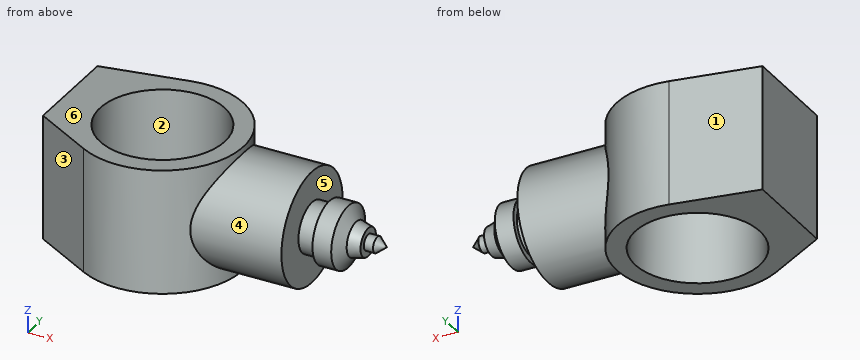
from build123d import *

# Parameters (mm, degrees)
IZIM1_R                          = 50
Y_KSEKLIK_EKSTR_ZYON1_DEPTH      = 50
Y_KSEKLIK_EKSTR_ZYON2_REACH      = 218.16
Y_KSEKLIK_EKSTR_ZYON2_END_RADIUS = 65
IZIM2_R                          = 45


with BuildPart() as part:
    # Çizim1 → Yükseklik-Ekstrüzyon1 (new, symmetric)
    with BuildSketch(Plane.XY):
        with BuildLine():
            Line((-80, -28.89070525), (-80, 51.10929475))
            Line((-80, 51.10929475), (-12, 63.882705015))
            ThreePointArc((-12, 63.882705015), (64.076421536, -10.918434095), (-32.479384713, -56.303548455))
            Line((-32.479384713, -56.303548455), (-80, -28.89070525))
        make_face()
        Circle(IZIM1_R, mode=Mode.SUBTRACT)
    extrude(amount=Y_KSEKLIK_EKSTR_ZYON1_DEPTH, both=True)

    # Yükseklik-Ekstrüzyon2: up to this cylinder (the profile starts outside it)
    y_kseklik_ekstr_zyon2_end = Plane(origin=(0, 0, 0), z_dir=(0, 0, -1)) * Cylinder(Y_KSEKLIK_EKSTR_ZYON2_END_RADIUS, 567.32, mode=Mode.PRIVATE)
    # Çizim2 → Yükseklik-Ekstrüzyon2 (add, up to the surface)
    with BuildSketch(Plane(origin=(120, 0, 0), x_dir=(0, 0, -1), z_dir=(1, 0, 0)), mode=Mode.PRIVATE) as y_kseklik_ekstr_zyon2_sk1:
        Circle(IZIM2_R)
    y_kseklik_ekstr_zyon2_tool1 = extrude(y_kseklik_ekstr_zyon2_sk1.sketch, amount=-Y_KSEKLIK_EKSTR_ZYON2_REACH, mode=Mode.PRIVATE) - y_kseklik_ekstr_zyon2_end
    add(y_kseklik_ekstr_zyon2_tool1.solids().sort_by_distance((120, 0, 0))[0])

    # Çizim3 → Döndür1 (revolve)
    with BuildSketch(Plane.XY, mode=Mode.PRIVATE) as d_nd_r1_sk:
        Polygon((164.385328123, -6.351150209), (172.385328123, -6.351150209), (180.109503873, 0), (120, 0), (120, -20), (134, -20), (134, -25), (149, -25), (155.385874648, -13.93934066), (165.04513291, -11.351150209), (165.04513291, -6.351150209), align=None)
    revolve(d_nd_r1_sk.sketch.rotate(Axis((0, 0, 0), (1, 0, 0)), 270), axis=Axis((0, 0, 0), (1, 0, 0)))


solid = part.part
Input: part model. Units: mm. Frame: model coordinates. Face numbers are marked on the shaded views. A direction names the side the tool comes from. Coordinates: 2 decimals unless noted, no trailing zeros. Order: outer loops, then holes, each group sorted by start corner. A loop starts at its lowest first (then second) coordinate and runs counter-clockwise, first axis right, second up. Notation, with made-up numbers: M 3,-39 L 37,-39 A22 cw 37,-33 Z; hole C -14,-33.5 d5. An arc over 180 degrees is marked long. Answer in a Markdown table with one row per item.
(1) Contact query for flat-ended pins moving along their axis: pin 1 Ø5 at (x, y) = (103.5, -34) entering from -Z; pin 2 Ø1.5 at (y, z) = (-44.5, -1) entering from +X; pin 3 Ø25 at (y, z) = (-3, -2.5) entering from +X; pin 4 Ø1.5 at (y, z) = (46.5, 20) entering from +X. Output: stop coordinate, or through.
Numbers:
| item | result |
|---|---|
| pin 1 | stops at z = -32.14 |
| pin 2 | stops at x = 120 |
| pin 3 | stops at x = 180.11 |
| pin 4 | stops at x = 46.17 |
(2) Section query C-C, the plane z = 34. Output: boundary loops of the cut face in (x, y).
Numbers:
| item | result |
|---|---|
| outline | M -80,-28.89 L -32.48,-56.3 A65 ccw 57.93,-29.48 L 120,-29.48 L 120,29.48 L 57.93,29.48 A65 ccw -12,63.88 L -80,51.11 Z; hole C 0,0 d100 |
(3) Section query A-A, the plane x = 0. Output: boundary loops of the cut face in (y, z).
Numbers:
| item | result |
|---|---|
| outline | M -65,-50 L -50,-50 L -50,50 L -65,50 Z; M 50,-50 L 65,-50 L 65,50 L 50,50 Z |
(4) Material intervals for line 1 (Y direction, x = 0, z = 5.5); line 2 (X direction, y = 10, z = -1.5); line 3 (X direction, y = -29.5, z = 25.5), sorted ascending. Write a range as [from, to].
Numbers:
| item | result |
|---|---|
| line 1 | y = [-65, -50], [50, 65] |
| line 2 | x = [-80, -48.99], [48.99, 165.05] |
| line 3 | x = [-78.94, -40.37], [40.37, 120] |
(5) Access query for the marked faces 4, 5 and 6. Directions: +Z, -Z, +X, -X, +Y, -Y. A direction counts if a zero-diameter tool reaches every point of the face in a straight line with its end or side. Return the directions, or none.
Numbers:
| item | result |
|---|---|
| face 4 | +X |
| face 5 | none |
| face 6 | +Z, +X, -X, +Y, -Y |
(6) Section query B-B, the plane y = -36. Output: boundary loops of the cut face in (x, z), plus the area to 3 significant figures.
Numbers:
| item | result |
|---|---|
| outline | M -67.68,-50 L -34.7,-50 L -34.7,50 L -67.68,50 Z; M 34.7,-50 L 54.12,-50 L 54.12,-27 L 120,-27 L 120,27 L 54.12,27 L 54.12,50 L 34.7,50 Z |
| area | 8,800 mm^2 |
(7) Section query D-D, the plane x = 58.5. Output: boundary loops of the cut face in (y, z), plus the area to 3 significant figures.
Numbers:
| item | result |
|---|---|
| outline | M -28.33,-50 L 28.33,-50 L 28.33,-34.96 A45 ccw 28.33,34.96 L 28.33,50 L -28.33,50 L -28.33,34.96 A45 ccw -28.33,-34.96 Z |
| area | 7,290 mm^2 |
(8) Draft query along Y for the marked faces 1, 2 and 3. Return one class per face: pulls with the +Y half, pulls with the -Y half, needs draft (parallel to the pull), parting line crosses it, or undercut.
Numbers:
| item | result |
|---|---|
| face 1 | pulls with the +Y half |
| face 2 | undercut |
| face 3 | pulls with the -Y half |
